The listing builds one solid part. Answer for the finished solid, in the listing's coordinates (mm). A direction names the side the tool comes from. Round coordinates to 2 decimals unless told otherwise and drop trailing zeros. Order: outer loops, then holes, each group sorted by start corner. A loop starts at its lowest first (then second) coordinate and runs counter-clockwise, first axis right, second up. Notation, with made-up numbers: (-38, -6) - (19, -6) arc R21 cw to (19, 5) - close; hole circle Ø1 at (24, -7). An arc over 180 degrees is marked (long way). Use CSV: the item, a comma, the result in double quotes. Start each with the question number.
Item 1: Straight lines are drawn through the part: line 1 along Y through (x, z) = (0, 10.25); line 2 along X through (y, z) = (-118, 8.75); line 3 along Z through (x, y) = (2, -64). For each, find the intervals that lie inside material, in ascending order. Write a range as [from, to].
Item 2: Determine the mould class of faces 6 (the cylindrical face through (4.85, -59.16, 14.25)), 7 (the flat face through (5, 3, 8)), 8 (the flat face through (-2, 1, 8)) for opening direction Y: +Y half, -Y half, draft (parallel to the pull), parting line (faces both ways), or undercut.
Item 3: Find section C-C, the plane y = -15. Give the vertices of the cut face in (x, z).
Item 4: Find section A-A, the plane x = 4.75. Give the vertices of the cut face in (y, z).
Item 5: Flat-ended cylindrical pins translate along their axes: P1, Ø6, axis at x = 1, y = -66, coming from the +Z side; P2, Ø1, axis at y = -42, z = 4.5, coming from the -X side; P3, Ø1.5, axis at x = 6.5, y = -96.5, coming from the +Z side. Find the tip coordinate at first contact, or state that the pin passes through.
Item 6: Find section B-B, the plane z = 4.25. Give the vertices of the cut face in (x, y), plus the area to 3 significant figures.
Item 7: For faces 1 (the flat face through (9.5, -59, 5)), 2 (the flat face through (5, -121, 16.25)), 3 (the flat face through (0, -59, 5)), 4 (the flat face through (11.5, 1, 8)), 5 (the flat face through (1.7, 0, 13.4)), determine the directions among +Z, -Z, +X, -X, +Y, -Y from which every point of the face is accessible in a straight line to the end or side of a thin tool.
```python
from build123d import *

# Parameters (mm, degrees)
BOSS_EXTRUDE1_DEPTH = 120
SKETCH8_W           = 13.5
SKETCH8_H           = 16.25
BOSS_EXTRUDE4_DEPTH = 3
SKETCH9_W           = 13.5
SKETCH9_H           = 16.25
BOSS_EXTRUDE5_DEPTH = 3


with BuildPart() as part:
    # Sketch5 → Boss-Extrude1 (new body)
    with BuildSketch(Plane(origin=(0, 0, 0), x_dir=(1, 0, 0), z_dir=(0, 1, 0))):
        with BuildLine():
            Line((0, 0), (9.5, 0))
            Line((9.5, 0), (9.5, -9.5))
            ThreePointArc((9.5, -9.5), (4.75, -14.25), (0, -9.5))
            Line((0, -9.5), (0, 0))
        make_face()
    extrude(amount=-BOSS_EXTRUDE1_DEPTH)

    # Sketch8 → Boss-Extrude4 (add)
    with BuildSketch(Plane.XZ.offset(120)):
        with Locations((4.75, 8.125)):
            Rectangle(SKETCH8_W, SKETCH8_H)
    extrude(amount=BOSS_EXTRUDE4_DEPTH)

    # Sketch9 → Boss-Extrude5 (add)
    with BuildSketch(Plane(origin=(0, 0, 0), x_dir=(1, 0, 0), z_dir=(0, 1, 0))):
        with Locations((4.75, -8.125)):
            Rectangle(SKETCH9_W, SKETCH9_H)
    extrude(amount=BOSS_EXTRUDE5_DEPTH)


solid = part.part
```
Worked out:
1,line 1,"y = [-123, -120], [0, 3]"
1,line 2,"x = [0, 9.5]"
1,line 3,"z = [0, 13.37]"
2,face 6,"undercut"
2,face 7,"+Y half"
2,face 8,"draft"
3,outline,"(0, 0) - (9.5, 0) - (9.5, 9.5) arc R4.75 ccw to (0, 9.5) - close"
4,outline,"(-123, 0) - (3, 0) - (3, 16.25) - (0, 16.25) - (0, 14.25) - (-120, 14.25) - (-120, 16.25) - (-123, 16.25) - close"
5,P1,"stops at z = 14.19"
5,P2,"stops at x = 0"
5,P3,"stops at z = 14.14"
6,outline,"(-2, -123) - (11.5, -123) - (11.5, -120) - (9.5, -120) - (9.5, 0) - (11.5, 0) - (11.5, 3) - (-2, 3) - (-2, 0) - (0, 0) - (0, -120) - (-2, -120) - close"
6,area,"1,220 mm²"
7,face 1,"+Z, -Z, +X"
7,face 2,"+Z, +X, -X, +Y, -Y"
7,face 3,"+Z, -Z, -X"
7,face 4,"+Z, -Z, +X, +Y, -Y"
7,face 5,"+Z"
